For this review, take the finished solid that the model builds, in its own axes (mm). Face numbers are marked on the shaded views. A direction names the side the tool comes from. Give positions to 0.01 mm unless a question says otherwise; leave off trailing zeros. Order: outer loops, then holes, each group sorted by start corner. A loop starts at its lowest first (then second) coordinate and runs counter-clockwise, first axis right, second up. Notation, with made-up numbers: (-21, 55) - (29, 55) arc R18 ccw to (29, 69) - close; hole circle Ø10 at (66, -23.75). An arc over 180 degrees is marked (long way). Put each result on its own line as item: value. Start each with the question number.
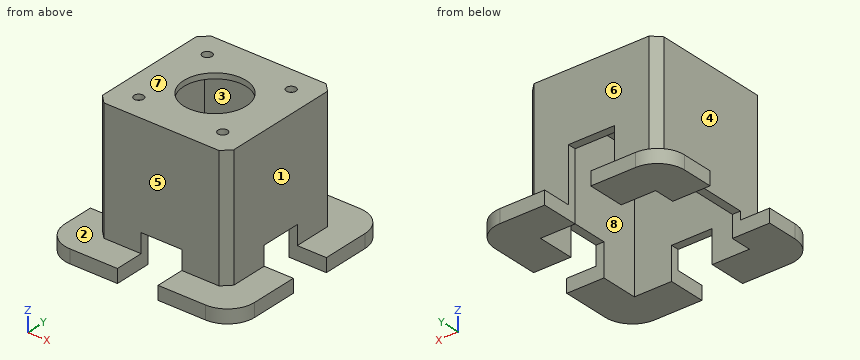
```python
from build123d import *

# Parameters (mm, degrees)
SKETCH_1_W          = 42.5
SKETCH_1_H          = 42.5
SKETCH_1_R          = 1.75
EXTRUDE_1_DEPTH     = 2
SKETCH_2_W          = 48.5
SKETCH_2_H          = 48.5
SKETCH_2_W_2        = 42.5
SKETCH_2_H_2        = 42.5
EXTRUDE_2_DEPTH     = 50
CHAMFER_1_SIZE      = 3
SKETCH_3_W          = 70
SKETCH_3_H          = 70
SKETCH_3_W_2        = 42.5
SKETCH_3_H_2        = 42.5
EXTRUDE_2_2_DEPTH   = 5
FILLET_1_R          = 10
CUT_EXTRUDE_2_REACH = 93.81
SKETCH_5_W          = 17
SKETCH_5_H          = 33.225295521
CUT_EXTRUDE_3_REACH = 93.81
SKETCH_6_W          = 17.032391735
SKETCH_6_H          = 27
SKETCH_7_R          = 11.5
CUT_EXTRUDE_4_DEPTH = 10
CUT_EXTRUDE_5_REACH = 93.81
SKETCH_9_W          = 15
SKETCH_9_H          = 14
CUT_EXTRUDE_6_REACH = 93.81
SKETCH_10_W         = 19.722222222
SKETCH_10_H         = 15


with BuildPart() as part:
    # 草图1 → 凸台-拉伸1 (new body)
    with BuildSketch(Plane.XY):
        Rectangle(SKETCH_1_W, SKETCH_1_H)
        with Locations((15.5, 15.5)):
            Circle(SKETCH_1_R, mode=Mode.SUBTRACT)
        with Locations((15.5, -15.5)):
            Circle(SKETCH_1_R, mode=Mode.SUBTRACT)
        with Locations((-15.5, -15.5)):
            Circle(SKETCH_1_R, mode=Mode.SUBTRACT)
        with Locations((-15.5, 15.5)):
            Circle(SKETCH_1_R, mode=Mode.SUBTRACT)
    extrude(amount=EXTRUDE_1_DEPTH)

    # 草图2 → Extrude 2 (add)
    with BuildSketch(Plane.XY.offset(2)):
        Rectangle(SKETCH_2_W, SKETCH_2_H)
        Rectangle(SKETCH_2_W_2, SKETCH_2_H_2, mode=Mode.SUBTRACT)
    extrude(amount=-EXTRUDE_2_DEPTH)

    # 倒角1
    chamfer_1_edges = [part.edges().sort_by_distance(p)[0] for p in [
        (-24.25, -24.25, -23),
        (-24.25, 24.25, -23),
        (24.25, 24.25, -23),
        (24.25, -24.25, -23),
    ]]
    chamfer(chamfer_1_edges, length=CHAMFER_1_SIZE)

    # 草图3 → Extrude 2 2 (add)
    with BuildSketch(Plane(origin=(0, 0, -48), x_dir=(-1, 0, 0), z_dir=(0, 0, -1))):
        Rectangle(SKETCH_3_W, SKETCH_3_H)
        Rectangle(SKETCH_3_W_2, SKETCH_3_H_2, mode=Mode.SUBTRACT)
    extrude(amount=-EXTRUDE_2_2_DEPTH)

    # 圆角1
    fillet_1_edges = [part.edges().sort_by_distance(p)[0] for p in [
        (35, -35, -45.5),
        (35, 35, -45.5),
        (-35, 35, -45.5),
        (-35, -35, -45.5),
    ]]
    fillet(fillet_1_edges, radius=FILLET_1_R)

    # 切除-拉伸2: up to this face of the body (flat: up to its plane)
    cut_extrude_2_end = Plane(part.part.faces().sort_by_distance((0, 21.25, -24))[0])
    # 草图5 → 切除-拉伸2 (cut, up to the picked face)
    with BuildSketch(Plane(origin=(0, 35, 0), x_dir=(1, 0, 0), z_dir=(0, 1, 0)), mode=Mode.PRIVATE) as cut_extrude_2_sk1:
        with Locations((0, 39.612647761)):
            Rectangle(SKETCH_5_W, SKETCH_5_H)
    cut_extrude_2_tool1 = split(extrude(cut_extrude_2_sk1.sketch, amount=-CUT_EXTRUDE_2_REACH, mode=Mode.PRIVATE), bisect_by=cut_extrude_2_end, keep=Keep.BOTH, mode=Mode.PRIVATE)
    add(cut_extrude_2_tool1.solids().sort_by(Axis((0, 35, -39.612648), (0, -1, 0)))[0], mode=Mode.SUBTRACT)

    # 切除-拉伸3: up to this face of the body (flat: up to its plane)
    cut_extrude_3_end = Plane(part.part.faces().sort_by_distance((-21.25, 0, -24))[0])
    # 草图6 → 切除-拉伸3 (cut, up to the picked face)
    with BuildSketch(Plane.ZY.offset(35), mode=Mode.PRIVATE) as cut_extrude_3_sk1:
        with Locations((-48.516195868, 0)):
            Rectangle(SKETCH_6_W, SKETCH_6_H)
    cut_extrude_3_tool1 = split(extrude(cut_extrude_3_sk1.sketch, amount=-CUT_EXTRUDE_3_REACH, mode=Mode.PRIVATE), bisect_by=cut_extrude_3_end, keep=Keep.BOTH, mode=Mode.PRIVATE)
    add(cut_extrude_3_tool1.solids().sort_by(Axis((-35, 0, -48.516196), (1, 0, 0)))[0], mode=Mode.SUBTRACT)

    # 草图7 → 切除-拉伸4 (cut)
    with BuildSketch(Plane.XY.offset(2)):
        Circle(SKETCH_7_R)
    extrude(amount=-CUT_EXTRUDE_4_DEPTH, mode=Mode.SUBTRACT)

    # 草图9 → 切除-拉伸5 (cut, up to next)
    with BuildSketch(Plane.XZ.offset(35), mode=Mode.PRIVATE) as cut_extrude_5_sk1:
        with Locations((0, -43)):
            Rectangle(SKETCH_9_W, SKETCH_9_H)
    cut_extrude_5_tool1 = extrude(cut_extrude_5_sk1.sketch, amount=-CUT_EXTRUDE_5_REACH, mode=Mode.PRIVATE) & part.part
    add(cut_extrude_5_tool1.solids().sort_by_distance((0, -35, -43))[0], mode=Mode.SUBTRACT)

    # 草图10 → 切除-拉伸6 (cut, up to next)
    with BuildSketch(Plane(origin=(35, 0, 0), x_dir=(0, 0, -1), z_dir=(1, 0, 0)), mode=Mode.PRIVATE) as cut_extrude_6_sk1:
        with Locations((45.861111111, 0)):
            Rectangle(SKETCH_10_W, SKETCH_10_H)
    cut_extrude_6_tool1 = extrude(cut_extrude_6_sk1.sketch, amount=-CUT_EXTRUDE_6_REACH, mode=Mode.PRIVATE) & part.part
    add(cut_extrude_6_tool1.solids().sort_by_distance((35, 0, -45.861111))[0], mode=Mode.SUBTRACT)


solid = part.part
```
1. Add section D-D, the plane z = -39. Give the boundary of the cut face in (x, y).
2. The part is to be moulded in two halves that separate along Y. For the marked faces 6, 7 and 8, say which applies: released by +Y, released by -Y, zero draft, split by the parting line, or undercut.
3. Add section B-B, the plane y = 15.5. Give the boundary of the cut face in (x, z).
4. Clearance check with flat-ended pins moving along their axes: pin 1 (3.5 mm diameter, centred on x = -1, y = 23.5, fed in from -Z); pin 2 (5 mm diameter, centred on y = 6.5, z = -42, fed in from -X); pin 3 (10 mm diameter, centred on x = 5, z = -22.5, fed in from -Y). State where each tip first meets the part, or that it passes through.
5. Tool access review of the marked faces 1, 2, 3, 4 and 5: name each direction out of +Z, -Z, +X, -X, +Y, -Y from which nothing blocks a thin tool from reaching the whole face with its end or side.
6. Add section A-A, the plane x = 0. Give the boundary of the cut face in (y, z).
7. Wall thickness on line 1 (Y direction, x = -15.5, z = 1.4); line 2 (X direction, y = -17, z = -11): over which ranges is each line inside the solid? List them lowest first. Write a range as from..to.
Found:
1. outline: (-24.25, -21.25) - (-21.25, -24.25) - (-7.5, -24.25) - (-7.5, -21.25) - (-21.25, -21.25) - (-21.25, 21.25) - (-8.5, 21.25) - (-8.5, 24.25) - (-21.25, 24.25) - (-24.25, 21.25) - close; (7.5, -24.25) - (21.25, -24.25) - (24.25, -21.25) - (24.25, -7.5) - (21.25, -7.5) - (21.25, -21.25) - (7.5, -21.25) - close; (8.5, 21.25) - (21.25, 21.25) - (21.25, 7.5) - (24.25, 7.5) - (24.25, 21.25) - (21.25, 24.25) - (8.5, 24.25) - close
2. face 6: released by +Y
2. face 7: zero draft
2. face 8: undercut
3. outline: (-35, -48) - (-21.25, -48) - (-21.25, 0) - (-17.25, 0) - (-17.25, 2) - (-24.25, 2) - (-24.25, -43) - (-35, -43) - close; (-13.75, 0) - (13.75, 0) - (13.75, 2) - (-13.75, 2) - close; (17.25, 0) - (21.25, 0) - (21.25, -48) - (35, -48) - (35, -43) - (24.25, -43) - (24.25, 2) - (17.25, 2) - close
4. pin 1: stops at z = -23
4. pin 2: stops at x = -24.25
4. pin 3: stops at y = -24.25
5. face 1: +Z, +X, +Y, -Y
5. face 2: +Z, -X, -Y
5. face 3: -Z
5. face 4: +Z, -X, +Y, -Y
5. face 5: +Z, +X, -X, -Y
6. outline: (-24.25, -36) - (-21.25, -36) - (-21.25, 0) - (-11.5, 0) - (-11.5, 2) - (-24.25, 2) - close; (11.5, 0) - (21.25, 0) - (21.25, -23) - (24.25, -23) - (24.25, 2) - (11.5, 2) - close
7. line 1: y = -24.25..-17.25, -13.75..13.75, 17.25..24.25
7. line 2: x = -24.25..-21.25, 21.25..24.25
